```python
from build123d import *

# Parameters (mm, degrees)
F0_W     = 100
F0_H     = 40
F1_DEPTH = 12
F2_W     = 16
F2_H     = 12
F3_DEPTH = 15
F4_W     = 16
F4_H     = 12
F5_DEPTH = 15
F6_R     = 15
F7_DEPTH = 40


with BuildPart() as f1:
    # F0 (on Top) → F1 (new body)
    with BuildSketch(Plane.XY):
        with Locations((50, 20)):
            Rectangle(F0_W, F0_H)
    extrude(amount=F1_DEPTH)

    # F2 (on face) → F3 (cut)
    with BuildSketch(Plane.YZ.offset(100)):
        with Locations((20, 6)):
            Rectangle(F2_W, F2_H)
    extrude(amount=-F3_DEPTH, mode=Mode.SUBTRACT)

    # F4 (on face) → F5 (cut)
    with BuildSketch(Plane(origin=(0, 0, 0), x_dir=(0, -1, 0), z_dir=(-1, 0, 0))):
        with Locations((-20, 6)):
            Rectangle(F4_W, F4_H)
    extrude(amount=-F5_DEPTH, mode=Mode.SUBTRACT)

    # F6 (on face) → F7 (join)
    with BuildSketch(Plane(origin=(0, 0, 0), x_dir=(1, 0, 0), z_dir=(0, 0, -1))):
        with BuildLine():
            ThreePointArc((58.422061, -40), (67.454528, -30.862784), (70.756012, -18.446086))
            ThreePointArc((70.756012, -18.446086), (68.634577, -8.367828), (62.63031, 0))
            Line((62.63031, 0), (28.881715, 0))
            ThreePointArc((28.881715, 0), (20.893229, -21.061805), (33.089963, -40))
            Line((33.089963, -40), (58.422061, -40))
        make_face()
        with Locations((45.756012, -18.446086)):
            Circle(F6_R, mode=Mode.SUBTRACT)
    extrude(amount=-F7_DEPTH)


solid = f1.part
```
Could you check a few things on this model? Use its own coordinates, in mm. A direction names the side the tool comes from. Round coordinates to 2 decimals unless told otherwise and drop trailing zeros. Write each loop counter-clockwise with the first axis right and the second up, starting at its lowest first coordinate (ties: lowest second). Pieces come first, ordered by that corner, then holes. Notation, with made-up numbers: M 1,57 L 27,57 A29 cw 27,90 Z; hole C 69.25,83 d2. An arc over 180 degrees is marked long. Answer in a Markdown table with one row per item. Add a question column.
Q1. Imagine slicing it at A-A (x = 88.5). Please give me the cut outline in (y, z), then the cut area to 3 significant figures.
Q2. Imagine slicing it at D-D (x = 51). Please give me the cut outline in (y, z).
Q3. If I drill on line 1 (Y direction, x = 8, z = 10.5); line 2 (Z direction, x = 46.5, y = 20); line 3 (X direction, y = 29, z = 21), over which ranges is the centre line in solid material (lowest first)? Write a range as from..to.
Q4. Imagine slicing it at C-C (y = 30). Please give me the cut outline in (x, z), then the cut area to 3 significant figures.
Q5. On a 3-axis mill with a long thin cutter (end or side, diameter ignored), from which of +Z, -Z, +X, -X, +Y, -Y can I reach the whole of each face in a straight line? I mean faces 5 (the flat face through (0, 6, 6)), 6 (the flat face through (93, 12, 6)), 7 (the cylindrical face through (30.77, 17.79, 25.8)), 8 (the flat face through (7, 12, 6)). Say none if no direction works.
Q6. If we mould it in two halves opening along X, with no side actions, what happens to faces 1 (the flat face through (100, 6, 6)), 2 (the flat face through (34, 29, 40)), 3 (the flat face through (46, 19, 12)), 4 (the cylindrical face through (20.86, 20.74, 25.8))? For each: +X half, -X half, draft (parallel to the pull), parting line (faces both ways), or undercut.
Q7. Imagine slicing it at B-B (z = 31.5). Please give me the cut outline in (x, y), then the cut area to 3 significant figures.
Q8. Will these pins go through, and if not, where does the flat tip stop? pin 1 Ø3.5 at (y, z) = (21, 8) entering from -X; pin 2 Ø3 at (y, z) = (15, 25.5) entering from +X; pin 3 Ø4 at (x, y) = (12.5, 33) entering from -Z; pin 4 Ø15 at (x, y) = (49.5, 22.5) entering from +Z.
Values:
| question | item | result |
|---|---|---|
| 1 | outline | M 0,0 L 12,0 L 12,12 L 0,12 Z; M 28,0 L 40,0 L 40,12 L 28,12 Z |
| 1 | area | 288 mm^2 |
| 2 | outline | M 0,0 L 40,0 L 40,40 L 32.5,40 L 32.5,12 L 4.39,12 L 4.39,40 L 0,40 Z |
| 3 | line 1 | 0..12, 28..40 |
| 3 | line 2 | 0..12 |
| 3 | line 3 | 23.09..35.1, 56.42..68.42 |
| 4 | outline | M 0,0 L 100,0 L 100,12 L 67.93,12 L 67.93,40 L 55.32,40 L 55.32,12 L 36.19,12 L 36.19,40 L 23.59,40 L 23.59,12 L 0,12 Z |
| 4 | area | 1,910 mm^2 |
| 5 | face 5 | +Z, -Z, -X, +Y, -Y |
| 5 | face 6 | +Z, -Z, +X |
| 5 | face 7 | +Z |
| 5 | face 8 | +Z, -Z, -X |
| 6 | face 1 | +X half |
| 6 | face 2 | draft |
| 6 | face 3 | undercut |
| 6 | face 4 | -X half |
| 7 | outline | M 28.88,0 L 62.63,0 A25 ccw 70.76,18.45 A25 ccw 58.42,40 L 33.09,40 A25 ccw Z; hole C 45.76,18.45 d30 |
| 7 | area | 1,050 mm^2 |
| 8 | pin 1 | x = 15 |
| 8 | pin 2 | x = 70.68 |
| 8 | pin 3 | z = 0 |
| 8 | pin 4 | z = 12 |
